Geometry check sheet. Reference: drawing and pictorial views, mm from the part's lowest x, y, z. A direction names the side the tool comes from. Round coordinates to 2 decimals unless told otherwise and drop trailing zeros. Order: outer loops, then holes, each group sorted by start corner. A loop starts at its lowest first (then second) coordinate and runs counter-clockwise, first axis right, second up.
(1) Set-up check for the marked faces 4, 5, 6 and 7: record each of +Z, -Z, +X, -X, +Y, -Y from which the full face is reachable in a straight line by a thin tool's end or side.
(2) Sectioned sample at A-A (y = 6). Record the boundary of the cut face in (x, z), plus the area to 3 significant figures.
(3) Material ranges on line 1 along Z through (x, y) = (1, 8.25); line 2 along Y through (x, z) = (6, 12.5); line 3 along Z through (x, y) = (6, 3.5), recorded low to high.
(4) Go/stop test with flat-tipped pins: pin 1 (4 mm diameter, centred on x = 5, z = 6.5, fed in from +Y); pin 2 (5 mm diameter, centred on y = 9, z = 4, fed in from -X); pin 3 (1.5 mm diameter, centred on y = 5.5, z = 12.5, fed in from +X). Record where each tip stops, or that it passes through.
(5) Release check for a two-part mould opening along Y. For the marked faces 1, 2 and 3 record: +Y half, -Y half, draft (parallel to the pull), parting line (faces both ways), or undercut.
(6) Sectioned sample at D-D (y = 4). Record the boundary of the cut face in (x, z), plus the area to 3 significant figures.
(7) Sectioned sample at C-C (z = 11.5). Record the boundary of the cut face in (x, y).
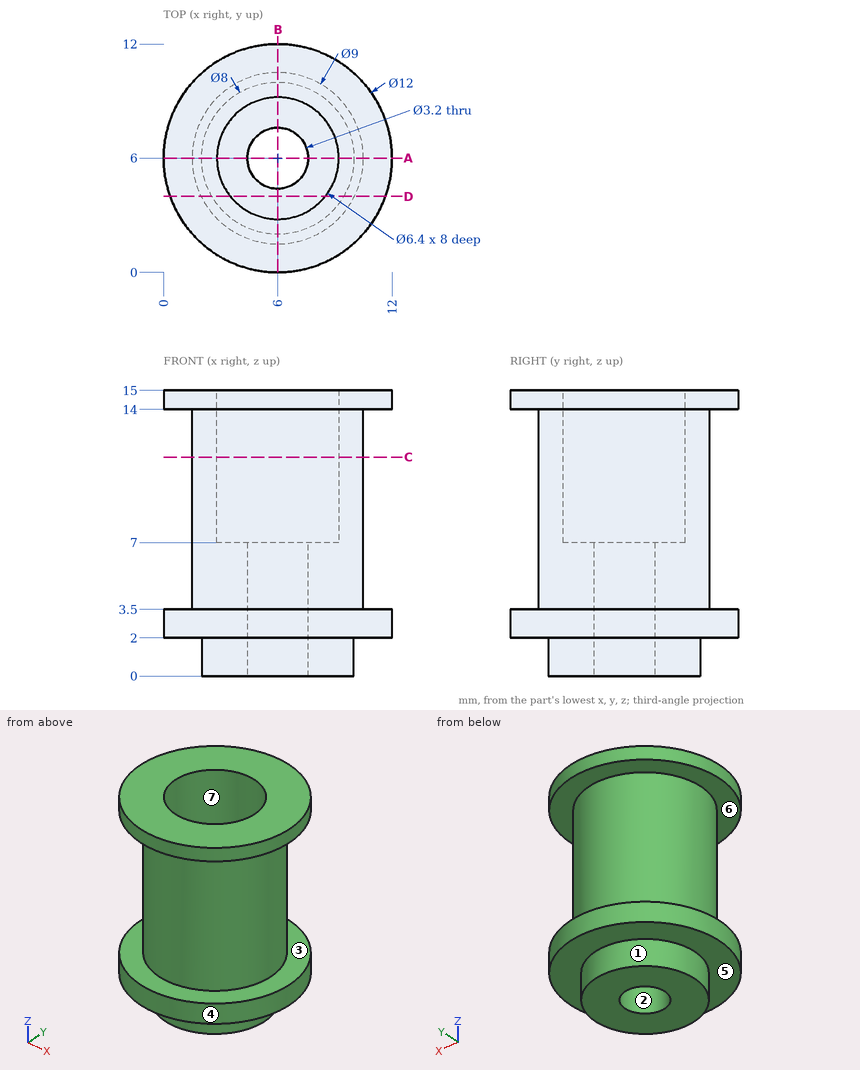
Answer below:
1. face 4: +Z, -Z
1. face 5: -Z
1. face 6: none
1. face 7: +Z
2. outline: (0, 2) - (2, 2) - (2, 0) - (4.4, 0) - (4.4, 7) - (2.8, 7) - (2.8, 15) - (0, 15) - (0, 14) - (1.5, 14) - (1.5, 3.5) - (0, 3.5) - close; (7.6, 0) - (10, 0) - (10, 2) - (12, 2) - (12, 3.5) - (10.5, 3.5) - (10.5, 14) - (12, 14) - (12, 15) - (9.2, 15) - (9.2, 7) - (7.6, 7) - close
2. area: 66.9 mm2
3. line 1: z = 2 to 3.5, 14 to 15
3. line 2: y = 1.5 to 2.8, 9.2 to 10.5
3. line 3: z = 0 to 7
4. pin 1: stops at y = 10.5
4. pin 2: stops at x = 0.03
4. pin 3: stops at x = 10.5
5. face 1: parting line
5. face 2: undercut
5. face 3: draft
6. outline: (0.34, 2) - (2.54, 2) - (2.54, 0) - (9.46, 0) - (9.46, 2) - (11.66, 2) - (11.66, 3.5) - (10.03, 3.5) - (10.03, 14) - (11.66, 14) - (11.66, 15) - (8.5, 15) - (8.5, 7) - (3.5, 7) - (3.5, 15) - (0.34, 15) - (0.34, 14) - (1.97, 14) - (1.97, 3.5) - (0.34, 3.5) - close
6. area: 86.8 mm2
7. outline: circle Ø9 at (6, 6); hole circle Ø6.4 at (6, 6)
